Check sheet for the modelled part. Datum: model origin and axes. Units: mm. A direction names the side the tool comes from. Round coordinates to 2 decimals unless told otherwise and drop trailing zeros. Write each loop counter-clockwise with the first axis right and the second up, starting at its lowest first coordinate (ties: lowest second). Pieces come first, ordered by that corner, then holes. Notation, with made-up numbers: M 82.25,12 L 121.25,12 A12 cw 121.25,21 Z; hole C 31,89 d5. An arc over 180 degrees is marked long. Put each result on its own line as item: value.
```python
from build123d import *

# Parameters (mm, degrees)
EXTRUDE_1_DEPTH     = 3
CUT_EXTRUDE_1_DEPTH = 3
SKETCH_3_R          = 1.5
CUT_EXTRUDE_2_DEPTH = 3
SKETCH_4_R          = 1.5
CUT_EXTRUDE_3_DEPTH = 4


with BuildPart() as part:
    # 草图1 → 凸台-拉伸1 (new body)
    with BuildSketch(Plane.XY):
        with BuildLine():
            Line((-53.903075976, 5), (42.782990351, 5))
            ThreePointArc((42.782990351, 5), (47.782990351, 0), (42.782990351, -5))
            Line((42.782990351, -5), (-51.223584051, -5))
            ThreePointArc((-51.223584051, -5), (-52.517679277, -5.170370869), (-53.723584051, -5.669872981))
            Line((-53.723584051, -5.669872981), (-94.717009649, -29.337438285))
            ThreePointArc((-94.717009649, -29.337438285), (-101.547136668, -27.507311266), (-99.717009649, -20.677184247))
            Line((-99.717009649, -20.677184247), (-56.403075976, 4.330127019))
            ThreePointArc((-56.403075976, 4.330127019), (-55.197171201, 4.829629131), (-53.903075976, 5))
        make_face()
    extrude(amount=EXTRUDE_1_DEPTH)

    # 草图2 → 切除-拉伸1 (cut)
    with BuildSketch(Plane.XY.offset(3)):
        with BuildLine():
            Line((-98.334747096, -22.771095042), (-72.598059837, -7.912011725))
            ThreePointArc((-72.598059837, -7.912011725), (-69.182829293, -8.82736459), (-70.098638571, -12.242472773))
            Line((-70.098638571, -12.242472773), (-96.083409035, -27.235527963))
            ThreePointArc((-96.083409035, -27.235527963), (-99.449240201, -26.132987403), (-98.334747096, -22.771095042))
        make_face()
    extrude(amount=-CUT_EXTRUDE_1_DEPTH, mode=Mode.SUBTRACT)

    # 草图3 → 切除-拉伸2 (cut)
    with BuildSketch(Plane.XY.offset(3)):
        with Locations((-31.303593391, 0)):
            Circle(SKETCH_3_R)
        with Locations((-41.303593391, 0)):
            Circle(SKETCH_3_R)
    extrude(amount=-CUT_EXTRUDE_2_DEPTH, mode=Mode.SUBTRACT)

    # 草图4 → 切除-拉伸3 (cut, through all)
    with BuildSketch(Plane(origin=(0, 0, 0), x_dir=(-1, 0, 0), z_dir=(0, 0, -1))):
        with Locations((-18.696406609, 0)):
            Circle(SKETCH_4_R)
        with Locations((-28.696406609, 0)):
            Circle(SKETCH_4_R)
    extrude(amount=-CUT_EXTRUDE_3_DEPTH, mode=Mode.SUBTRACT)


solid = part.part
```
1. Cross-section at B-B (y = 0). Enter the section's corners in (x, z), then the cut area to 3 significant figures.
Computed values:
outline: M -63.9,0 L -42.8,0 L -42.8,3 L -63.9,3 Z; M -39.8,0 L -32.8,0 L -32.8,3 L -39.8,3 Z; M -29.8,0 L 17.2,0 L 17.2,3 L -29.8,3 Z; M 20.2,0 L 27.2,0 L 27.2,3 L 20.2,3 Z; M 30.2,0 L 47.78,0 L 47.78,3 L 30.2,3 Z
area: 299 mm2
2. Cross-section at C-C (y = -19). Enter the section's corners in (x, z).
Computed values:
outline: M -96.81,0 L -91.8,0 L -91.8,3 L -96.81,3 Z; M -81.81,0 L -76.81,0 L -76.81,3 L -81.81,3 Z
3. Release check for a two-part mould opening along Y. For faces 1 (the flat face through (-21, -3, 3)), 2 (the cylindrical face through (-101.49, -27.6, 1.48)), 3 (the cylindrical face through (17.266, 0.451, 1.479)) record: +Y half, -Y half, draft (parallel to the pull), parting line (faces both ways), or undercut.
Computed values:
face 1: draft
face 2: parting line
face 3: undercut
4. Scan lines: probe 1 along Y at (x, z) = (-93, 2.45); probe 2 along X at (y, z) = (-11, 0.75); probe 3 along Y at (x, z) = (-11.5, 2.05). Record each from-to range of solid material in increasing order.
Computed values:
probe 1: y = -28.35 to -25.46, -19.69 to -16.8
probe 2: x = -82.96 to -77.95, -69.02 to -62.96
probe 3: y = -5 to 5
5. Access from +Z, -Z, +X, -X, +Y, -Y to the whole of each face (thin tool, end or side, straight path). Record for faces 4 (the flat face through (-82.909, -19.634, 1.521)), 5 (the flat face through (-4, -5, 1)), 6 (the cylindrical face through (47.78, 0.11, 1.48)).
Computed values:
face 4: +Z, -Z
face 5: +Z, -Z, +X, -Y
face 6: +Z, -Z, +X
6. Cross-section at A-A (z = 1.2). Enter the section's corners in (x, y), then the cut area to 3 significant figures.
Computed values:
outline: M -99.72,-20.68 A5 ccw -94.72,-29.34 L -53.72,-5.67 A5 cw -51.22,-5 L 42.78,-5 A5 ccw 42.78,5 L -53.9,5 A5 ccw -56.4,4.33 Z; hole M -98.33,-22.77 A2.5 ccw long -96.08,-27.24 L -70.1,-12.24 A2.5 ccw -72.6,-7.91 Z; hole C -41.3,0 d3; hole C -31.3,0 d3; hole C 18.7,0 d3; hole C 28.7,0 d3
area: 1,350 mm2
7. Cross-section at D-D (x = -89.5). Enter the section's corners in (y, z).
Computed values:
outline: M -26.33,0 L -23.44,0 L -23.44,3 L -26.33,3 Z; M -17.67,0 L -14.78,0 L -14.78,3 L -17.67,3 Z
8. Depth check by flat-ended pin: pin 1 Ø1.5 at (y, z) = (-23.5, 2.5) entering from -X; pin 2 Ø1 at (y, z) = (-19.5, 2) entering from -X; pin 3 Ø1.8 at (x, y) = (-41.3, 0) entering from +Z. Enter the tip coordinate at first touch or a pass-through.
Computed values:
pin 1: stops at x = -102.16
pin 2: stops at x = -98.54
pin 3: passes through
